Geometry check sheet. Reference: the model listing, model coordinates, mm. Face numbers are marked on the shaded views. A direction names the side the tool comes from. Give positions to 0.01 mm unless a question says otherwise; leave off trailing zeros. Loops run counter-clockwise (first coordinate to the right, second up) from the corner with the lowest first, then second, coordinate; pieces in that order, holes last. Notation, with made-up numbers: (35.5, 86) - (86.5, 86) arc R21 cw to (86.5, 90) - close; hole circle Ø5 at (42.25, 16.25). An arc over 180 degrees is marked (long way). One line per question, with ' | ' between items. Start each with the question number.
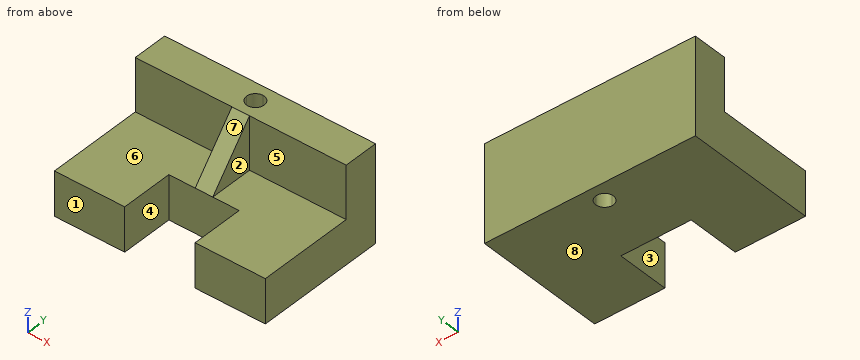
from build123d import *

# Parameters (mm, degrees)
SKETCH_1_W          = 120
SKETCH_1_H          = 75
EXTRUDE_1_DEPTH     = 25
SKETCH_2_W          = 40
SKETCH_2_H          = 25
CUT_EXTRUDE_1_DEPTH = 30
SKETCH_3_W          = 120
SKETCH_3_H          = 20
EXTRUDE_2_DEPTH     = 30
EXTRUDE_START       = -55
EXTRUDE_3_DEPTH     = 10
CUT_EXTRUDE_2_DEPTH = 152.822264507


with BuildPart() as part:
    # Эскиз1 → Бобышка-Вытянуть1 (new body)
    with BuildSketch(Plane.XY):
        with Locations((60, -37.5)):
            Rectangle(SKETCH_1_W, SKETCH_1_H)
    extrude(amount=EXTRUDE_1_DEPTH)

    # Эскиз2 → Вырез-Вытянуть1 (cut)
    with BuildSketch(Plane.XZ.offset(75)):
        with Locations((60, 12.5)):
            Rectangle(SKETCH_2_W, SKETCH_2_H)
    extrude(amount=-CUT_EXTRUDE_1_DEPTH, mode=Mode.SUBTRACT)

    # Эскиз3 → Бобышка-Вытянуть2 (add)
    with BuildSketch(Plane.XY.offset(25)):
        with Locations((60, -10)):
            Rectangle(SKETCH_3_W, SKETCH_3_H)
    extrude(amount=EXTRUDE_2_DEPTH)

    # Эскиз5 → Бобышка-Вытянуть3 (add)
    with BuildSketch(Plane(origin=(120, 0, 0), x_dir=(0, 0, -1), z_dir=(1, 0, 0)).offset(EXTRUDE_START)):
        Polygon((-55, -20), (-25, -45), (-25, -20), align=None)
    extrude(amount=-EXTRUDE_3_DEPTH)

    # Эскиз6 → Вырез-Вытянуть2 (cut, through all)
    with BuildSketch(Plane.XY.offset(55)):
        with BuildLine():
            ThreePointArc((55, -10), (56.464466094, -13.535533906), (60, -15))
            Line((60, -15), (60, -10))
            Line((60, -10), (55, -10))
        make_face()
        with BuildLine():
            Line((60, -10), (60, -15))
            ThreePointArc((60, -15), (63.535533906, -13.535533906), (65, -10))
            Line((65, -10), (60, -10))
        make_face()
        with BuildLine():
            Line((55, -10), (60, -10))
            Line((60, -10), (60, -5))
            ThreePointArc((60, -5), (56.464466094, -6.464466094), (55, -10))
        make_face()
        with BuildLine():
            Line((60, -5), (60, -10))
            Line((60, -10), (65, -10))
            ThreePointArc((65, -10), (63.535533906, -6.464466094), (60, -5))
        make_face()
    extrude(amount=-CUT_EXTRUDE_2_DEPTH, mode=Mode.SUBTRACT)


solid = part.part
(1) Section check D-D, the plane y = -43. Record the boundary of the cut face in (x, z).
(2) Depth check by flat-ended pin: pin 1 Ø7.5 at (y, z) = (-59, 13) entering from -X; pin 2 Ø9 at (x, z) = (31.5, 43.5) entering from -Y; pin 3 Ø12.5 at (x, z) = (57.5, 11.5) entering from -Y; pin 4 Ø12.5 at (y, z) = (-34, 32.5) entering from -X. Enter the tip coordinate at first touch or a pass-through.
(3) Mould release check, pull along X, two halves, no side actions. Record for the marked faces 1, 2 and 3: pulls with the +X half, pulls with the -X half, needs draft (parallel to the pull), parting line crosses it, or undercut.
(4) Tool access check on the marked faces 4, 5, 6, 7 and 8. Record the directions out of +Z, -Z, +X, -X, +Y, -Y that give a thin tool (end or side, any length) a straight path to the whole face; none if there is none.
(5) Section check C-C, the plane x = 62.5. Record the boundary of the cut face in (y, z), and give its area (3 significant figures).
(6) Section check A-A, the plane y = -60.5. Record the boundary of the cut face in (x, z), and give its area (3 significant figures).
(7) Material ranges on line 1 (X direction, y = -49.5, z = 24); line 2 (Z direction, x = 5.5, y = -29); line 3 (Y direction, x = 79, z = 14), recorded low to high.
(8) Section check B-B, the plane z = 8. Record the boundary of the cut face in (x, y).
Numbers:
1) outline: (0, 0) - (120, 0) - (120, 25) - (65, 25) - (65, 27.4) - (55, 27.4) - (55, 25) - (0, 25) - close
2) pin 1: x = 0 | pin 2: y = -20 | pin 3: y = -45 | pin 4: x = 55
3) face 1: needs draft | face 2: pulls with the +X half | face 3: undercut
4) face 4: +Z, -Z, -Y | face 5: +Z, +X, -Y | face 6: +Z, -X, -Y | face 7: +Z, +X, -X, -Y | face 8: -Z, +X, -X, +Y, -Y
5) outline: (-45, 0) - (-14.33, 0) - (-14.33, 55) - (-20, 55) - (-45, 25) - close; (-5.67, 0) - (0, 0) - (0, 55) - (-5.67, 55) - close | area: 1,620 mm^2
6) outline: (0, 0) - (40, 0) - (40, 25) - (0, 25) - close; (80, 0) - (120, 0) - (120, 25) - (80, 25) - close | area: 2,000 mm^2
7) line 1: 0 to 40, 80 to 120 | line 2: 0 to 25 | line 3: -45 to 0
8) outline: (0, -75) - (40, -75) - (40, -45) - (80, -45) - (80, -75) - (120, -75) - (120, 0) - (0, 0) - close; hole circle Ø10 at (60, -10)
